For this review, take the finished solid that the model builds, in its own axes (mm). A direction names the side the tool comes from. Round coordinates to 2 decimals unless told otherwise and drop trailing zeros. Order: outer loops, then holes, each group sorted by start corner. A loop starts at its lowest first (then second) coordinate and runs counter-clockwise, first axis right, second up. Notation, with made-up numbers: M 85.5,82.5 L 123.5,82.5 A7 ccw 123.5,92.5 Z; hole C 22.5,-25.75 d7. An arc over 180 degrees is marked long. Answer as a JSON object with one key per item and string values.
Autodesk Inventor part; units mm, degrees
ref_plane "YZ Plane" through (0, 0, 0) normal (1, 0, 0) x (0, 1, 0)
ref_plane "XZ Plane" through (0, 0, 0) normal (0, 1, 0) x (-1, 0, 0)
ref_plane "XY Plane" through (0, 0, 0) normal (0, 0, 1) x (1, 0, 0)
sketch "Sketch1" plane through (0, 0, 0) normal (1, 0, 0) x (0, 1, 0)
  line L0 (0, 0) -> (58, 0)
  line L1 (58, -250) -> (0, -250)
  line L2 (78, -6) -> (78, -21)
  line L3 (78, -21) -> (58, -21)
  line L4 (58, -21) -> (58, -125)
  line L5 (78, -21) -> (78, -6)
  line L6 (78, -21) -> (78, -6)
  line L7 (78, -229) -> (58, -229)
  line L8 (58, -229) -> (58, -125)
  line L9 (78, -244) -> (58, -250)
  line L10 (78, -244) -> (78, -229)
  line L11 (0, 0) -> (0, -62)
  line L12 (0, -62) -> (20, -62)
  line L13 (20, -75) -> (0, -75)
  arc A0 (20, -75) -> (20, -62) centre (20, -68.5) ccw
  line L14 (78, -6) -> (78, -21)
  line L15 (78, -229) -> (78, -244)
  line L16 (0, -250) -> (0, -75)
  line L17 (0, -62) -> (0, 0)
  line L18 (58, 0) -> (0, 0)
  line L19 (0, 0) -> (0, -62)
  line L20 (0, -62) -> (20, -62)
  arc A1 (20, -75) -> (20, -62) centre (20, -68.5) ccw
  line L21 (20, -75) -> (0, -75)
  line L22 (0, -75) -> (0, -250)
  line L23 (0, -250) -> (58, -250)
  line L24 (58, 0) -> (0, 0)
  line L25 (78, -6) -> (58, 0)
  dimension "d8" = 62
  dimension "d10" = 13
  dimension "d21" = 15
  dimension "d22" = 15
extrude "Extrusion2" add sketch "Sketch1" along normal blind 17
sketch "Sketch2" plane through (0, 0, 0) normal (-1, 0, 0) x (0, 0, 1)
  line L0 (-75, 0) -> (-250, 0)
  line L1 (-229, 42) -> (-238, 42)
  line L2 (-238, 42) -> (-238, 10)
  line L3 (-75, 0) -> (-250, 0)
  line L4 (-229, 42) -> (-179, 42)
  line L5 (-179, 42) -> (-179, 56)
  line L6 (-238, 10) -> (-125, 10)
  line L7 (-21, 42) -> (-12, 42)
  line L8 (-12, 42) -> (-12, 10)
  line L9 (-21, 42) -> (-71, 42)
  line L10 (-71, 42) -> (-71, 56)
  line L11 (-12, 10) -> (-125, 10)
  line L12 (-179, 56) -> (-71, 56)
  point P0 (-229, 58)
  dimension "d14" = 16
  dimension "d15" = 9
  dimension "d23" = 32
extrude "Extrusion3" cut sketch "Sketch2" against normal blind 15
properties part number "Right Side" material "Steel"
1) Add section D-D on x = 2.5. State the section outline as (y, z) points.
Geometry check:
{"outline": "M 0,-250 L 58,-250 L 78,-244 L 78,-229 L 58,-229 L 58,-21 L 78,-21 L 78,-6 L 58,0 L 0,0 L 0,-62 L 10,-62 L 10,-12 L 42,-12 L 42,-71 L 56,-71 L 56,-179 L 42,-179 L 42,-238 L 10,-238 L 10,-75 L 0,-75 Z"}
2) Insertion check: P1, Ø5, axis at x = 5.5, y = 63.5, coming from the +Z side; P2, Ø1, axis at x = 7, y = 61, coming from the +Z side; P3, Ø8.5, axis at x = 9.5, z = -107, coming from the +Y side. Each pin has a flat end and moves straight along its axis. Give the tip position at first contact, or say it passes through.
Geometry check:
{"P1": "stops at z = -0.9", "P2": "stops at z = -0.75", "P3": "stops at y = 58"}
3) Mouldability with a two-part tool opening along Y and no side actions: class faces 1 (the flat face through (7, 49, -71)), 2 (the flat face through (8, 0, -164)), 3 (the flat face through (7, 26, -12)), 4 (the flat face through (7, 42, -41)) as +Y half, -Y half, draft (parallel to the pull), parting line (faces both ways), or undercut.
Geometry check:
{"face 1": "draft", "face 2": "-Y half", "face 3": "undercut", "face 4": "undercut"}
4) Add section A-A on y = 17.5. State the section outline as (x, z) points, and give its area (3 significant figures).
Geometry check:
{"outline": "M 0,-250 L 17,-250 L 17,-75 L 15,-75 L 15,-238 L 0,-238 Z; M 0,-12 L 15,-12 L 15,-62 L 17,-62 L 17,0 L 0,0 Z", "area": "834 mm²"}
5) Add section B-B on z = -45.5. State the section outline as (x, y) points, and give its area (3 significant figures).
Geometry check:
{"outline": "M 0,0 L 17,0 L 17,58 L 0,58 L 0,42 L 15,42 L 15,10 L 0,10 Z", "area": "506 mm²"}
6) Machinability: for faces 5 (the flat face through (7, 10, -155)), 6 (the flat face through (17, 30, -123)), 7 (the flat face through (8, 6, -75)), 8 (the flat face through (8, 68, -3)), 9 (the flat face through (8, 58, -124)), which of the approach directions +Z, -Z, +X, -X, +Y, -Y give a long, thin tool a straight path to every point of the face, cutting with its end or side? Answer none if there is none.
Geometry check:
{"face 5": "-X", "face 6": "+Z, -Z, +X, +Y, -Y", "face 7": "+X, -X, -Y", "face 8": "+Z, +X, -X, +Y", "face 9": "+X, -X, +Y"}
7) For L1, parallel to Z at x = 11.5, y = 35.5; L2, parallel to Y at x = 9.5, z = -224.5; L3, parallel to Y at x = 3.75, z = -87, list the stretches that pass through material, from the lowest coordinate up.
Geometry check:
{"L1": "z = -250 to -238, -12 to 0", "L2": "y = 0 to 10, 42 to 58", "L3": "y = 0 to 10, 56 to 58"}
8) Add section C-C on y = 37.5. State the section outline as (x, z) points.
Geometry check:
{"outline": "M 0,-250 L 17,-250 L 17,0 L 0,0 L 0,-12 L 15,-12 L 15,-238 L 0,-238 Z"}
